Build history of the part. All positions in model axes, mm. A direction names the side the tool comes from. Round coordinates to 2 decimals unless told otherwise and drop trailing zeros. Loops run counter-clockwise (first coordinate to the right, second up) from the corner with the lowest first, then second, coordinate; pieces in that order, holes last. Notation, with made-up numbers: (15.25, 11.5) - (72.25, 11.5) arc R25 cw to (72.25, 43.5) - close; hole circle Ø7 at (-22.75, -28.5). An arc over 180 degrees is marked (long way). Answer as CSV lines item,"result". Start each with the question number.
```python
from build123d import *

# Parameters (mm, degrees)
SKETCH_1_R          = 13
SKETCH_1_R_2        = 6
SKETCH_1_R_3        = 1.5
EXTRUDE_1_DEPTH     = 3
SKETCH_2_R          = 7.4
SKETCH_2_R_2        = 6
EXTRUDE_2_DEPTH     = 1
CUT_EXTRUDE_START   = -41
CUT_EXTRUDE_1_DEPTH = 41


with BuildPart() as part:
    # 草图1 → 凸台-拉伸1 (new body)
    with BuildSketch(Plane.XY):
        Circle(SKETCH_1_R)
        Circle(SKETCH_1_R_2, mode=Mode.SUBTRACT)
        with Locations((-7.071067812, 7.071067812)):
            Circle(SKETCH_1_R_3, mode=Mode.SUBTRACT)
        with Locations((7.071067812, 7.071067812)):
            Circle(SKETCH_1_R_3, mode=Mode.SUBTRACT)
        with Locations((7.071067812, -7.071067812)):
            Circle(SKETCH_1_R_3, mode=Mode.SUBTRACT)
        with Locations((-7.071067812, -7.071067812)):
            Circle(SKETCH_1_R_3, mode=Mode.SUBTRACT)
    extrude(amount=EXTRUDE_1_DEPTH)

    # 草图2 → 凸台-拉伸2 (add)
    with BuildSketch(Plane.XY.offset(3)):
        Circle(SKETCH_2_R)
        Circle(SKETCH_2_R_2, mode=Mode.SUBTRACT)
    extrude(amount=EXTRUDE_2_DEPTH)

    # 草图3 → 切除-拉伸1 (cut)
    with BuildSketch(Plane.XY.offset(3).offset(CUT_EXTRUDE_START)):
        with BuildLine():
            Line((-8.220315878, 10.071067812), (8.220315878, 10.071067812))
            ThreePointArc((8.220315878, 10.071067812), (0, 13), (-8.220315878, 10.071067812))
        make_face()
        with BuildLine():
            Line((10.071067812, 8.220315878), (10.071067812, -8.220315878))
            ThreePointArc((10.071067812, -8.220315878), (13, 0), (10.071067812, 8.220315878))
        make_face()
        with BuildLine():
            Line((8.220315878, -10.071067812), (-8.220315878, -10.071067812))
            ThreePointArc((-8.220315878, -10.071067812), (0, -13), (8.220315878, -10.071067812))
        make_face()
        with BuildLine():
            Line((-10.071067812, -8.220315878), (-10.071067812, 8.220315878))
            ThreePointArc((-10.071067812, 8.220315878), (-13, 0), (-10.071067812, -8.220315878))
        make_face()
    extrude(amount=CUT_EXTRUDE_1_DEPTH, mode=Mode.SUBTRACT)


solid = part.part
```
Q1. Two-plate mould, pull along Y, no slides. Class faces 1 (the cylindrical face through (8.502, 7.522, 1.479)), 2 (the cylindrical face through (9.205, 9.179, 1.479)), 3 (the cylindrical face through (-1.604, -7.224, 3.493)): released by +Y, released by -Y, zero draft, split by the parting line, or undercut.
Q2. Band-saw the part on A-A, the plane x = 0. List the corners of the cut face in (y, z).
Q3. Tool access for faces 4 (the flat face through (-5, 7, 3)), 5 (the cylindrical face through (-9.205, -9.179, 1.479)): list every direction of +Z, -Z, +X, -X, +Y, -Y with a clear straight run to the whole face (end or side of a thin tool).
Q4. Band-saw the part on C-C, the plane z = 0.45. List the corners of the cut face in (x, y).
Q5. Pin check, flat tips, straight feed: pin 1 Ø5 at (x, y) = (-7.07, 7.07) entering from +Z; pin 2 Ø10 at (x, y) = (-4.5, 3.5) entering from +Z. Stop position of each tip, or through.
Q6. Wall check: probe 1 along X at (y, z) = (7, 0.75); probe 2 along Y at (x, z) = (-8, 0.5); probe 3 along X at (y, z) = (-7.75, 1). Give the ranges that are in metal, low to high. Write a range as [from, to].
Reported:
1,face 1,"undercut"
1,face 2,"released by +Y"
1,face 3,"split by the parting line"
2,outline,"(-10.07, 0) - (-6, 0) - (-6, 4) - (-7.4, 4) - (-7.4, 3) - (-10.07, 3) - close; (6, 0) - (10.07, 0) - (10.07, 3) - (7.4, 3) - (7.4, 4) - (6, 4) - close"
3,face 4,"+Z"
3,face 5,"+Z, -Z, -X, -Y"
4,outline,"(-10.07, -8.22) arc R13 ccw to (-8.22, -10.07) - (8.22, -10.07) arc R13 ccw to (10.07, -8.22) - (10.07, 8.22) arc R13 ccw to (8.22, 10.07) - (-8.22, 10.07) arc R13 ccw to (-10.07, 8.22) - close; hole circle Ø3 at (-7.07, -7.07); hole circle Ø3 at (-7.07, 7.07); hole circle Ø12 at (0, 0); hole circle Ø3 at (7.07, -7.07); hole circle Ø3 at (7.07, 7.07)"
5,pin 1,"stops at z = 3"
5,pin 2,"stops at z = 4"
6,probe 1,"x = [-10.07, -8.57], [-5.57, 5.57], [8.57, 10.07]"
6,probe 2,"y = [-10.07, -8.25], [-5.89, 5.89], [8.25, 10.07]"
6,probe 3,"x = [-10.07, -8.41], [-5.73, 5.73], [8.41, 10.07]"
